Geometry check sheet. Reference: the model listing, model coordinates, mm. Face numbers are marked on the shaded views. A direction names the side the tool comes from. Coordinates: 2 decimals unless noted, no trailing zeros. Order: outer loops, then holes, each group sorted by start corner. A loop starts at its lowest first (then second) coordinate and runs counter-clockwise, first axis right, second up. Notation, with made-up numbers: M 20.25,36 L 27.25,36 A23 cw 27.25,74 Z; hole C -37.75,78 d6. An arc over 180 degrees is marked long. One line per item, written item: value. Start each with the question number.
1) Sectioned sample at A-A, the plane x = 23. Enter the section's corners in (y, z).
2) Thickness scan on L1, parallel to Y at x = 57, z = 0; L2, parallel to X at y = 7.5, z = -4; L3, parallel to Z at x = 37.5, y = 0.25. Record the ranges inside material, lowest first. Write a range as from..to.
3) Access from +Z, -Z, +X, -X, +Y, -Y to the whole of each face (thin tool, end or side, straight path). Record for the marked faces 1 and 2.
4) Go/stop test with flat-tipped pins: P1, Ø3, axis at y = 6.5, z = 5, coming from the +X side; P2, Ø2, axis at x = 41, y = 1, coming from the -Z side; P3, Ø6, axis at x = 44.5, z = -4, coming from the -Y side. Record where each tip stops, or that it passes through.
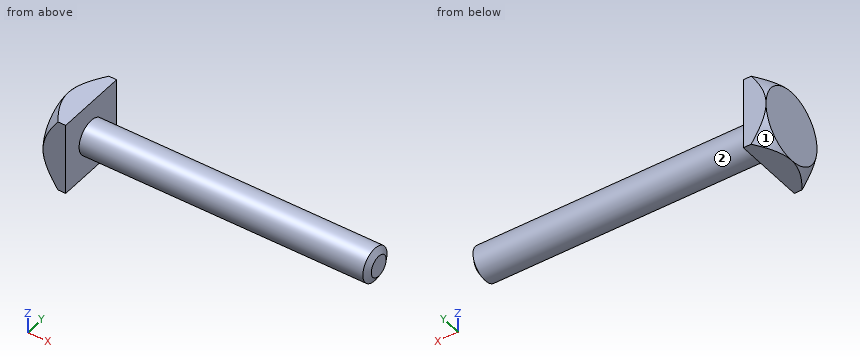
```python
from build123d import *

# Parameters (mm, degrees)
SKETCH1_W           = 19
SKETCH1_H           = 19
BOSS_EXTRUDE1_DEPTH = 6
SKETCH2_R           = 4.5
BOSS_EXTRUDE2_DEPTH = 76
CHAMFER1_SIZE       = 1
CHAMFER1_SIZE2      = 1.732050808
SKETCH3_OUTSIDE_W   = 58.258
SKETCH3_OUTSIDE_H   = 58.258
SKETCH3_OUTSIDE_R   = 9.5
CUT_EXTRUDE1_DEPTH  = 10
CUT_EXTRUDE1_DRAFT  = -45


with BuildPart() as part:
    # Sketch1 → Boss-Extrude1 (new body)
    with BuildSketch(Plane(origin=(0, 0, 0), x_dir=(0, 0, -1), z_dir=(1, 0, 0))):
        Rectangle(SKETCH1_W, SKETCH1_H)
    extrude(amount=BOSS_EXTRUDE1_DEPTH)

    # Sketch2 → Boss-Extrude2 (add)
    with BuildSketch(Plane(origin=(6, 0, 0), x_dir=(0, 0, -1), z_dir=(1, 0, 0))):
        with Locations(Location((0, 0, 0), (0, 0, 180))):  # turned: the seam where the file's is
            Circle(SKETCH2_R)
    extrude(amount=BOSS_EXTRUDE2_DEPTH)

    # Chamfer1
    chamfer1_edges = [part.edges().sort_by_distance(p)[0] for p in [
        (82, 0, -4.5),
    ]]
    chamfer1_side = [part.faces().sort_by_distance(p)[0] for p in [
        (44, 0, -4.5),
    ]]
    chamfer(chamfer1_edges, length=CHAMFER1_SIZE, length2=CHAMFER1_SIZE2, reference=chamfer1_side[0])


with BuildPart() as cut_extrude1_tool:
    # Sketch3 outside → Cut-Extrude1 (with draft: the straight prism first)
    with BuildSketch(Plane.ZY):
        Rectangle(SKETCH3_OUTSIDE_W, SKETCH3_OUTSIDE_H)
        Circle(SKETCH3_OUTSIDE_R, mode=Mode.SUBTRACT)
    extrude(amount=-CUT_EXTRUDE1_DEPTH)
    # Cut-Extrude1: the draft: its side faces are tilted about the plane it starts from
    cut_extrude1_sides = [cut_extrude1_tool.faces().sort_by_distance(p)[0] for p in [
        (5, -29.129, 0),
        (5, 0, 29.129),
        (5, 29.129, 0),
        (5, 0, -29.129),
        (5, 0, -9.5),
    ]]
    draft(cut_extrude1_sides, Plane.ZY, CUT_EXTRUDE1_DRAFT)


with BuildPart() as part_1:
    add(part.part)

    # Cut-Extrude1: cut by cut_extrude1_tool
    add(cut_extrude1_tool.part, mode=Mode.SUBTRACT)


solid = part_1.part
```
Final values:
1. outline: C 0,0 d9
2. L1: y = -4.5..4.5
2. L2: x = 0..6
2. L3: z = -4.49..4.49
3. face 1: -Z, -X, +Y
3. face 2: +X
4. P1: stops at x = 6
4. P2: stops at z = -4.5
4. P3: stops at y = -4.39
